from build123d import *

# Parameters (mm, degrees)
SKETCH_1_R          = 12.5
EXTRUDE_1_DEPTH     = 30
SKETCH_3_R          = 1.65
CUT_EXTRUDE_1_DEPTH = 4
SKETCH_4_R          = 6
EXTRUDE_2_DEPTH     = 2
SKETCH_5_R          = 2
EXTRUDE_3_DEPTH     = 10
FILLET_1_R          = 2


with BuildPart() as part:
    # 草图1 → 凸台-拉伸1 (new body)
    with BuildSketch(Plane.XY):
        Circle(SKETCH_1_R)
    extrude(amount=EXTRUDE_1_DEPTH)

    # 草图3 → 切除-拉伸1 (cut)
    with BuildSketch(Plane.XY.offset(30)):
        with Locations((-9, 0)):
            Circle(SKETCH_3_R)
        with Locations((9, 0)):
            Circle(SKETCH_3_R)
    extrude(amount=-CUT_EXTRUDE_1_DEPTH, mode=Mode.SUBTRACT)

    # 草图4 → 凸台-拉伸2 (add)
    with BuildSketch(Plane.XY.offset(30)):
        Circle(SKETCH_4_R)
    extrude(amount=EXTRUDE_2_DEPTH)

    # 草图5 → 凸台-拉伸3 (add)
    with BuildSketch(Plane.XY.offset(32)):
        Circle(SKETCH_5_R)
    extrude(amount=EXTRUDE_3_DEPTH)

    # 圆角1
    fillet_1_edges = [part.edges().sort_by_distance(p)[0] for p in [
        (-12.5, 0, 0),
    ]]
    fillet(fillet_1_edges, radius=FILLET_1_R)


solid = part.part
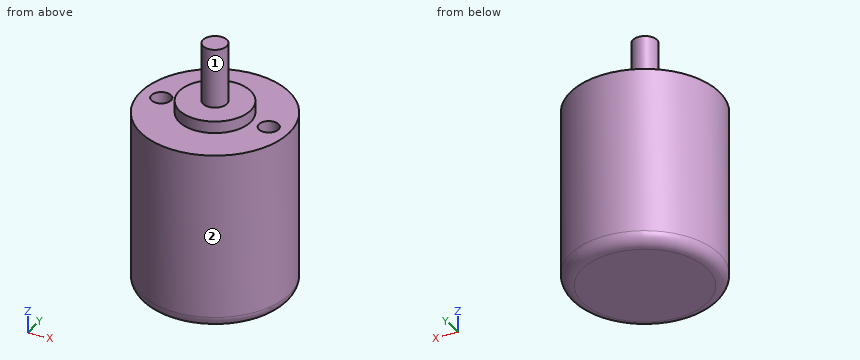
Source: CAD feature listing. Evaluate the final solid. Frame: model axes, mm. Face numbers are marked on the shaded views. A direction names the side the tool comes from. Give positions to 0.01 mm unless a question says otherwise; leave off trailing zeros. Loops run counter-clockwise (first coordinate to the right, second up) from the corner with the lowest first, then second, coordinate; pieces in that order, holes last. Notation, with made-up numbers: (54.25, -35) -> (77.25, -35) arc R26 cw to (77.25, -16) -> close; hole circle Ø4 at (67, 17.5). An arc over 180 degrees is marked (long way). Use a Markdown table: item, result. Add a question column.
1) Line query: line 1 along Z through (x, y) = (-8.25, -4.5); line 2 along Z through (x, y) = (-2.75, 1.75); line 3 along Y through (x, z) = (-9, 28.95). Output: solid intervals per line, ascending. Write a range as [from, to].
2) Section query B-B, the plane z = 27. Return the cut outline in (x, y), then the cut area to 3 significant figures.
3) First-contact query: pin 1 (1 mm diameter, centred on x = 5, y = -0.5, fed in from +Z); pin 2 (2.5 mm diameter, centred on x = 9.5, y = 0.5, fed in from +Z); pin 3 (8 mm diameter, centred on y = 7.5, z = 4.5, fed in from -X). Flat tips, straight axial feed; report the tip coordinate or a pass-through.
4) Reachability of the marked faces 1 and 2 from +Z, -Z, +X, -X, +Y, -Y: full face, straight path, thin tool, end or side. Return the list, or none.
5) Section query C-C, the plane x = 0. Return the cut outline in (y, z), then the cut area to 3 significant figures.
6) Section query D-D, the plane z = 18. Return the cut outline in (x, y), then the cut area to 3 significant figures.
7) Section query A-A, the plane y = 0. Return the cut outline in (x, z), then the cut area to 3 significant figures.
Numbers:
| question | item | result |
|---|---|---|
| 1 | line 1 | z = [0, 30] |
| 1 | line 2 | z = [0, 32] |
| 1 | line 3 | y = [-8.67, -1.65], [1.65, 8.67] |
| 2 | outline | circle Ø25 at (0, 0); hole circle Ø3.3 at (-9, 0); hole circle Ø3.3 at (9, 0) |
| 2 | area | 474 mm2 |
| 3 | pin 1 | stops at z = 32 |
| 3 | pin 2 | stops at z = 30 |
| 3 | pin 3 | stops at x = -12 |
| 4 | face 1 | +Z |
| 4 | face 2 | +Z, -Z |
| 5 | outline | (-12.5, 2) arc R2 ccw to (-10.5, 0) -> (10.5, 0) arc R2 ccw to (12.5, 2) -> (12.5, 30) -> (6, 30) -> (6, 32) -> (2, 32) -> (2, 42) -> (-2, 42) -> (-2, 32) -> (-6, 32) -> (-6, 30) -> (-12.5, 30) -> close |
| 5 | area | 812 mm2 |
| 6 | outline | circle Ø25 at (0, 0) |
| 6 | area | 491 mm2 |
| 7 | outline | (-12.5, 2) arc R2 ccw to (-10.5, 0) -> (10.5, 0) arc R2 ccw to (12.5, 2) -> (12.5, 30) -> (10.65, 30) -> (10.65, 26) -> (7.35, 26) -> (7.35, 30) -> (6, 30) -> (6, 32) -> (2, 32) -> (2, 42) -> (-2, 42) -> (-2, 32) -> (-6, 32) -> (-6, 30) -> (-7.35, 30) -> (-7.35, 26) -> (-10.65, 26) -> (-10.65, 30) -> (-12.5, 30) -> close |
| 7 | area | 786 mm2 |
